Work out the finished part from the listing and answer in its coordinate system (mm). A direction names the side the tool comes from. Round coordinates to 2 decimals unless told otherwise and drop trailing zeros. Loops run counter-clockwise (first coordinate to the right, second up) from the corner with the lowest first, then second, coordinate; pieces in that order, holes last. Notation, with made-up numbers: M -21,59 L 36,59 A13 ccw 36,81 Z; hole C 81,66.5 d10. An arc over 180 degrees is marked long. One line per item, written item: value.
```python
from build123d import *

# Parameters (mm, degrees)
CUT_EXTRUDE_1_DEPTH = 6
SKETCH_3_R          = 1.5
CUT_EXTRUDE_2_DEPTH = 5


with BuildPart() as part:
    # 草图1 → 旋转1 (revolve)
    with BuildSketch(Plane.XY):
        Polygon((0, 0), (2.5, 0), (2.5, -15), (1.5, -15), (1.5, -23), (0, -23), align=None)
    revolve(axis=Axis((0, 9.186035128, 0), (0, -1, 0)))

    # 草图2 → 切除-拉伸1 (cut)
    with BuildSketch(Plane(origin=(0, 0, 0), x_dir=(1, 0, 0), z_dir=(0, 1, 0))):
        with BuildLine():
            Line((-2, 1.5), (2, 1.5))
            ThreePointArc((2, 1.5), (0, 2.5), (-2, 1.5))
        make_face()
    extrude(amount=-CUT_EXTRUDE_1_DEPTH, mode=Mode.SUBTRACT)

    # 草图3 → 切除-拉伸2 (cut, through all)
    with BuildSketch(Plane(origin=(0, 0, -1.5), x_dir=(-1, 0, 0), z_dir=(0, 0, -1))):
        with Locations((0, -2.5)):
            Circle(SKETCH_3_R)
    extrude(amount=-CUT_EXTRUDE_2_DEPTH, mode=Mode.SUBTRACT)


solid = part.part
```
1) For faces 1 (the face through (0, -6, -2)), 2 (the face through (0, -23, 0)), 3 (the face through (-1.5, -19.06, 0.07)), determine the directions among +Z, -Z, +X, -X, +Y, -Y from which every point of the face is accessible in a straight line to the end or side of a thin tool.
Check values:
face 1: -Z, +X, -X, +Y
face 2: +Z, -Z, +X, -X, -Y
face 3: -Y
2) Find the intervals of material crossed by probe 1 along Y at (x, z) = (0, 0); probe 2 along X at (y, z) = (-2.5, -0.15); probe 3 along Y at (x, z) = (-1, 1.95), in increasing order. Write a range as from..to.
Check values:
probe 1: -23..-4, -1..0
probe 2: -2.5..-1.5, 1.5..2.5
probe 3: -15..-3.62, -1.38..0
3) Each of these flat-tipped pins is pushed along its axis until it touches: pin 1 (3 mm diameter, centred on y = -9.5, z = -0.5, fed in from +X); pin 2 (3 mm diameter, centred on x = -1, y = -3.5, fed in from -Z); pin 3 (2.5 mm diameter, centred on x = 0, y = -2.5, fed in from +Z) (3 decimals). Where does it stop, or does it pass through?
Check values:
pin 1: x = 2.5
pin 2: z = -1.5
pin 3: through
4) The mould has two halves that part along X. Classify faces 4 (the face through (0, -4.3, -1.5)), 5 (the face through (1.34, -9.27, 2.11)), 6 (the face through (-1.43, -2.05, 0.47)): +X half, -X half, draft (parallel to the pull), parting line (faces both ways), or undercut.
Check values:
face 4: draft
face 5: parting line
face 6: undercut
5) Find section A-A (x = 0). Give the vertices of the cut face in (y, z).
Check values:
outline: M -23,-1.5 L -15,-1.5 L -15,-2.5 L -6,-2.5 L -6,-1.5 L -4,-1.5 L -4,2.5 L -15,2.5 L -15,1.5 L -23,1.5 Z; M -1,-1.5 L 0,-1.5 L 0,2.5 L -1,2.5 Z
6) Find section B-B (y = -2.5). Give the vertices of the cut face in (x, z).
Check values:
outline: M -2,-1.5 L -1.5,-1.5 L -1.5,2 A2.5 ccw Z; M 1.5,-1.5 L 2,-1.5 A2.5 ccw 1.5,2 Z
7) Find section D-D (y = -9). Give the vertices of the cut face in (x, z).
Check values:
outline: C 0,0 d5
8) Find section C-C (z = 0). Give the vertices of the cut face in (x, y).
Check values:
outline: M -2.5,-15 L -1.5,-15 L -1.5,-23 L 1.5,-23 L 1.5,-15 L 2.5,-15 L 2.5,0 L -2.5,0 Z; hole C 0,-2.5 d3
